Can you work these out from the drawing? Everything is in mm from the part's minimum corner. A direction names the side the tool comes from. Round coordinates to 2 decimals unless told otherwise and drop trailing zeros. Answer as a JSON object with one key per item and string values.
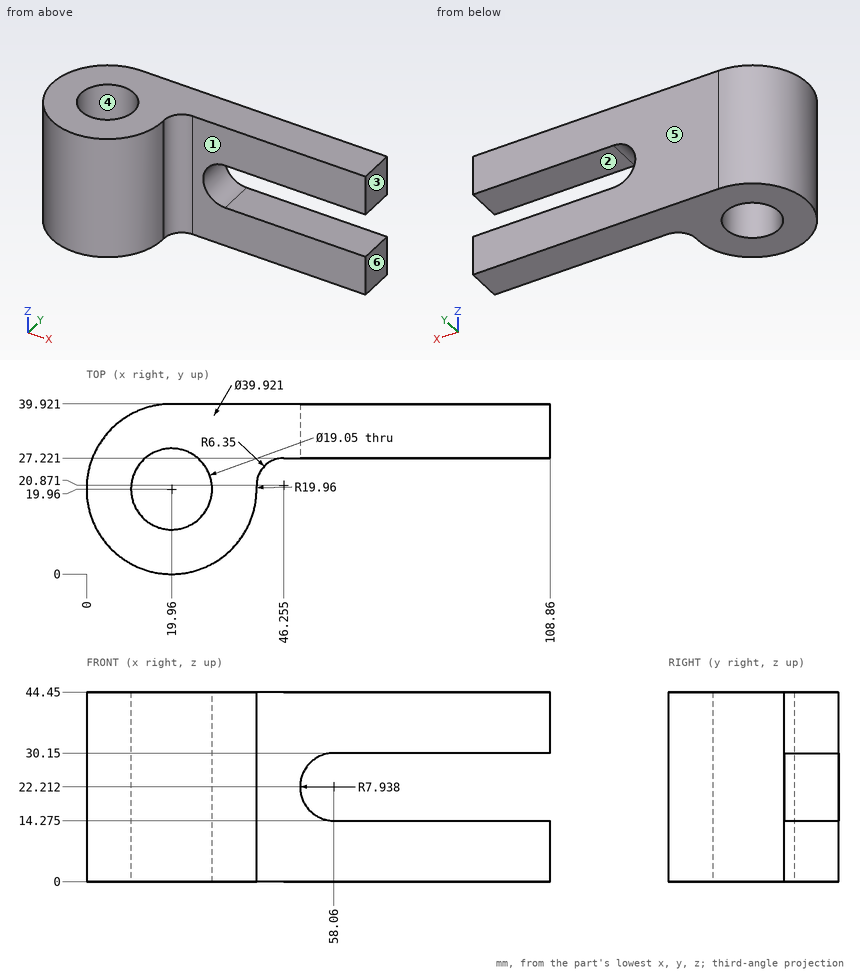
1. If I drill on L1, parallel to Y at x = 67, z = 42; L2, parallel to X at y = 14, z = 26.5; L3, parallel to Y at x = 21, z = 13, over which ranges is the centre line in solid material (lowest first)? Write a range as [from, to].
Responses:
{"L1": "[27.22, 39.92]", "L2": "[0.91, 12.53], [27.39, 39.01]", "L3": "[0.03, 10.49], [29.43, 39.92]"}
2. For the marked faces 1, 2 and 3, which set-ups out of +Z, -Z, +X, -X, +Y, -Y let a thin tool reach every point of the face, with its end or its side?
Responses:
{"face 1": "+Z, -Z, +X, -Y", "face 2": "+X, +Y, -Y", "face 3": "+Z, -Z, +X, +Y, -Y"}
3. For P1, Ø2, axis at y = 17.5, z = 24.5, coming from the +X side; P2, Ø2, axis at y = 35, z = 17, coming from the -X side; P3, Ø4, axis at y = 11.5, z = 27.5, coming from the +X side; P4, Ø11.5, axis at x = 19.96, y = 19.96, coming from the +Z side, each with a flat end and sliding along its axis, tell me the tip position at first contact or that it passes through.
Responses:
{"P1": "x = 39.87", "P2": "x = 5.77", "P3": "x = 38.85", "P4": "through"}
4. Thinking about a two-plate mould opening in Y: for the marked faces 4, 5 and 6, which applies, pulls with the +Y half, pulls with the -Y half, needs draft (parallel to the pull), parting line crosses it, or undercut?
Responses:
{"face 4": "undercut", "face 5": "pulls with the +Y half", "face 6": "needs draft"}
